```python
from build123d import *

# Parameters (mm, degrees)
F0_W     = 20
F0_H     = 20
F1_DEPTH = 20
F2_T     = -1
F4_D     = 1


with BuildPart() as f1:
    # F0 (on Top) → F1 (new body)
    with BuildSketch(Plane.XY):
        with Locations((8.472297, -16.565783)):
            Rectangle(F0_W, F0_H)
    extrude(amount=F1_DEPTH)

    # F2
    f2_openings = [f1.faces().sort_by_distance(p)[0] for p in [
        (8.472297, -16.565783, 20),
    ]]
    offset(amount=F2_T, openings=f2_openings)

    # F4 (through all)
    with Locations(Plane(origin=(0, 0, 0), x_dir=(1, 0, 0), z_dir=(0, 0, -1))):
        with Locations((14.472297, 10.565783), (8.472297, 10.565783), (2.472297, 10.565783), (2.472297, 16.565783), (8.472297, 16.565783), (14.472297, 16.565783), (14.472297, 22.565783), (8.472297, 22.565783), (2.472297, 22.565783)):
            Hole(F4_D / 2)


solid = f1.part
```
Work out the finished part from the listing and answer in its coordinate system (mm). A direction names the side the tool comes from. Coordinates: 2 decimals unless noted, no trailing zeros. Write each loop counter-clockwise with the first axis right and the second up, starting at its lowest first coordinate (ties: lowest second). Pieces come first, ordered by that corner, then holes. Notation, with made-up numbers: (11, -15) - (34, -15) arc R23 ccw to (34, 11) - close; hole circle Ø7 at (-36.75, 10). An arc over 180 degrees is marked (long way). Answer as a JSON object with one key per item and string values.
Q1. For a pull along Y with two mould halves and no side action, classify faces 1 (the flat face through (6, -16, 0)), 2 (the flat face through (8, -6.566, 10)), 3 (the cylindrical face through (14.54, -23.06, 0.51)) as pulls with the +Y half, pulls with the -Y half, needs draft (parallel to the pull), parting line crosses it, or undercut.
Results list:
{"face 1": "needs draft", "face 2": "pulls with the +Y half", "face 3": "undercut"}
Q2. Find section D-D (x = 14.5). Write down the section's boundary in (y, z), plus the area to 3 significant figures.
Results list:
{"outline": "(-26.57, 0) - (-23.07, 0) - (-23.07, 1) - (-25.57, 1) - (-25.57, 20) - (-26.57, 20) - close; (-22.07, 0) - (-17.07, 0) - (-17.07, 1) - (-22.07, 1) - close; (-16.07, 0) - (-11.07, 0) - (-11.07, 1) - (-16.07, 1) - close; (-10.07, 0) - (-6.57, 0) - (-6.57, 20) - (-7.57, 20) - (-7.57, 1) - (-10.07, 1) - close", "area": "55.0 mm^2"}
Q3. Find section B-B (x = 7.5). Write down the section's boundary in (y, z), plus the area to 3 significant figures.
Results list:
{"outline": "(-26.57, 0) - (-6.57, 0) - (-6.57, 20) - (-7.57, 20) - (-7.57, 1) - (-25.57, 1) - (-25.57, 20) - (-26.57, 20) - close", "area": "58.0 mm^2"}
Q4. Given pin 1 Ø1 at (x, y) = (4, -18) entering from +Z, flat-ended and moving along its own axis, determine where the tip first touches the part or whether it passes through.
Results list:
{"pin 1": "stops at z = 1"}
Q5. Which of the six approach directions +Z, -Z, +X, -X, +Y, -Y give full straight-line access (tool end or side, diameter ignored) to faces 4 (the flat face through (8, -18, 1)), 5 (the cylindrical face through (2.54, -23.06, 0.51))?
Results list:
{"face 4": "+Z", "face 5": "+Z, -Z"}
Q6. Consider L1, parallel to X at y = -7.75, z = 2.5; L2, parallel to Y at x = 5.25, z = 5.25; L3, parallel to Z at x = 13.75, y = -10.5. Determine where each line is inside the solid, lowest interval first. Write a range as from..to.
Results list:
{"L1": "x = -1.53..-0.53, 17.47..18.47", "L2": "y = -26.57..-25.57, -7.57..-6.57", "L3": "z = 0..1"}
Q7. Find section A-A (z = 17). Write down the section's boundary in (x, y).
Results list:
{"outline": "(-1.53, -26.57) - (18.47, -26.57) - (18.47, -6.57) - (-1.53, -6.57) - close; hole (-0.53, -25.57) - (17.47, -25.57) - (17.47, -7.57) - (-0.53, -7.57) - close"}
Q8. Find section C-C (y = -14). Write down the section's boundary in (x, z).
Results list:
{"outline": "(-1.53, 0) - (18.47, 0) - (18.47, 20) - (17.47, 20) - (17.47, 1) - (-0.53, 1) - (-0.53, 20) - (-1.53, 20) - close"}
